Build history of the part. All positions in model axes, mm. A direction names the side the tool comes from. Round coordinates to 2 decimals unless told otherwise and drop trailing zeros. Loops run counter-clockwise (first coordinate to the right, second up) from the corner with the lowest first, then second, coordinate; pieces in that order, holes last. Notation, with made-up numbers: (15.5, 58) - (48.5, 58) arc R21 cw to (48.5, 82) - close; hole circle Ø4 at (-26.5, 7). An arc over 180 degrees is marked (long way). Put each result on its own line as item: value. Start each with the question number.
from build123d import *

# Parameters (mm, degrees)
F1_DEPTH = 2
F2_R     = 0.5
F3_R     = 0.5


with BuildPart() as f1:
    # F0 (on Top) → F1 (new body)
    with BuildSketch(Plane.XY):
        Polygon((3.36771, 4.635255), (0, 15), (-3.36771, 4.635255), (-14.265848, 4.635255), (-5.449069, -1.77051), (-8.816779, -12.135255), (0, -5.72949), (8.816779, -12.135255), (5.449069, -1.77051), (14.265848, 4.635255), align=None)
    extrude(amount=F1_DEPTH)

    # F2
    f2_edges = [f1.edges().sort_by_distance(p)[0] for p in [
        (0, 15, 1),
        (-14.265848, 4.635255, 1),
        (14.265848, 4.635255, 1),
        (8.816779, -12.135255, 1),
        (-8.816779, -12.135255, 1),
    ]]
    fillet(f2_edges, radius=F2_R)

    # F3
    f3_edges = [f1.edges().sort_by_distance(p)[0] for p in [
        (0, -5.72949, 1),
        (5.449069, -1.77051, 1),
        (3.36771, 4.635255, 1),
        (-3.36771, 4.635255, 1),
        (-5.449069, -1.77051, 1),
    ]]
    fillet(f3_edges, radius=F3_R)


solid = f1.part
Item 1: Slice it at C-C (y = 6). Give the cut face in (x, z).
Item 2: Slice it at B-B (x = 0). Give the cut face in (y, z), plus the area to 3 significant figures.
Item 3: Slice it at A-A (z = 0.9). Give the cut face in (x, y), plus the area to 3 significant figures.
Item 4: Drill centre lines: probe 1 along X at (y, z) = (-8.25, 0.15); probe 2 along X at (y, z) = (-5, 1.05); probe 3 along Y at (x, z) = (-4.75, 0.1). Where is each one in solid material? Low to high. Write a range as [from, to].
Item 5: Drop a flat-ended pin along its axis: pin 1 Ø1 at (x, y) = (2.5, -8.5) entering from +Z. Give the stop position or say it passes through.
Item 6: Two-plate mould, pull along X, no slides. Class faces 1 (the flat face through (-3.98, -8.62, 0.99)), 2 (the flat face through (3.88, -8.55, 0.99)), 3 (the cylindrical face through (13.2, 4.3, 1)), 4 (the flat face through (0, 1, 2)): pulls with the +X half, pulls with the -X half, needs draft (parallel to the pull), parting line crosses it, or undercut.
Item 7: Which spindle directions (+Z, -Z, +X, -X, +Y, -Y) get a long thin tool onto all of the face, cutting with end or side? Do faces 5 (the flat face through (8, 4.635, 1)), 6 (the flat face through (9.33, 1.05, 0.99)), 7 (the flat face through (-8, 4.635, 1)), 8 (the flat face through (-9.4, 1.1, 1)). Say none if no direction does.
Computed values:
1. outline: (-2.92, 0) - (2.92, 0) - (2.92, 2) - (-2.92, 2) - close
2. outline: (-5.85, 0) - (13.88, 0) - (13.88, 2) - (-5.85, 2) - close
2. area: 39.5 mm^2
3. outline: (-13.02, 3.73) - (-5.74, -1.56) arc R0.5 cw to (-5.56, -2.12) - (-8.34, -10.67) arc R0.5 ccw to (-7.57, -11.23) - (-0.29, -5.94) arc R0.5 cw to (0.29, -5.94) - (7.57, -11.23) arc R0.5 ccw to (8.34, -10.67) - (5.56, -2.12) arc R0.5 cw to (5.74, -1.56) - (13.02, 3.73) arc R0.5 ccw to (12.73, 4.64) - (3.73, 4.64) arc R0.5 cw to (3.26, 4.98) - (0.48, 13.54) arc R0.5 ccw to (-0.48, 13.54) - (-3.26, 4.98) arc R0.5 cw to (-3.73, 4.64) - (-12.73, 4.64) arc R0.5 ccw to start
3. area: 250 mm^2
4. probe 1: x = [-7.55, -3.47], [3.47, 7.55]
4. probe 2: x = [-6.5, 6.5]
4. probe 3: y = [-9.18, 4.64]
5. pin 1: passes through
6. face 1: undercut
6. face 2: undercut
6. face 3: pulls with the +X half
6. face 4: needs draft
7. face 5: +Z, -Z, +X, +Y
7. face 6: +Z, -Z, +X
7. face 7: +Z, -Z, -X, +Y
7. face 8: +Z, -Z, -X
